For this review, take the finished solid that the model builds, in its own axes (mm). Give positions to 0.01 mm unless a question says otherwise; leave off trailing zeros. Order: outer loops, then holes, each group sorted by start corner. A loop starts at its lowest first (then second) coordinate and runs counter-clockwise, first axis right, second up. Notation, with made-up numbers: (61.25, 62) - (97.25, 62) arc R17 ccw to (97.25, 66) - close; hole circle Ø6 at (-35, -13.5). An arc over 180 degrees is marked (long way). Use a Markdown table: item, result. Add a question column.
1) We need section D-D on z = -60. Write out the cut boundary in (x, y), then the cut area to 3 significant figures.
2) Clearance check with flat-ended pins moving along their axes: P1, Ø0.9, axis at x = 84.5, y = 1.5, coming from the -Z side; P2, Ø1, axis at x = -97.5, y = 1, coming from the +Z side; P3, Ø0.9, axis at x = 87, y = 1, coming from the +Z side; P4, Ø2.5, axis at x = -60, z = 45, coming from the +Y side. State where each tip first meets the part, or that it passes through.
3) Wall thickness on L1, parallel to X at y = 0.25, z = 61; L2, parallel to Z at x = -60, y = 2; L3, parallel to X at y = 0.7, z = 15: over which ranges is each line inside the solid? List them lowest first.
4) We need section C-C on y = 1.3. Give the number of separate pieces and of enclosed holes in the cut face, then the cut area to 3 significant figures.
5) We need section B-B on z = 83.5. Write out the cut boundary in (x, y), then the cut area to 3 significant figures.
6) We need section A-A on z = 0. Write out the cut boundary in (x, y).
```python
from build123d import *

# Parameters (mm, degrees)
BOSS_EXTRUDE1_OUTLINE_R   = 150
BOSS_EXTRUDE1_OUTLINE_R_2 = 1.55
BOSS_EXTRUDE1_OUTLINE_W   = 30
BOSS_EXTRUDE1_OUTLINE_H   = 68
BOSS_EXTRUDE1_OUTLINE_R_3 = 2.25
BOSS_EXTRUDE1_DEPTH       = 3
SKETCH3_W                 = 5
SKETCH3_H                 = 63.96
SKETCH3_W_2               = 4
SKETCH3_H_2               = 6
CUT_EXTRUDE1_DEPTH        = 10


# Read off the part's stored shape, not the designer's step: Boss-Extrude1
with BuildPart() as part:
    # Boss-Extrude1 outline → Boss-Extrude1 (new body)
    with BuildSketch(Plane(origin=(0, 0, 0), x_dir=(1, 0, 0), z_dir=(0, 1, 0))):
        Circle(BOSS_EXTRUDE1_OUTLINE_R)
        with Locations((-60, -94)):
            Circle(BOSS_EXTRUDE1_OUTLINE_R_2, mode=Mode.SUBTRACT)
        with BuildLine():
            Line((-25.85, -95.55), (-31.95, -95.55))
            ThreePointArc((-31.95, -95.55), (-33.5, -94), (-31.95, -92.45))
            Line((-31.95, -92.45), (-25.85, -92.45))
            ThreePointArc((-25.85, -92.45), (-24.3, -94), (-25.85, -95.55))
        make_face(mode=Mode.SUBTRACT)
        with Locations((-89, -71)):
            Rectangle(BOSS_EXTRUDE1_OUTLINE_W, BOSS_EXTRUDE1_OUTLINE_H, mode=Mode.SUBTRACT)
        with Locations((-60, -45)):
            Circle(BOSS_EXTRUDE1_OUTLINE_R_2, mode=Mode.SUBTRACT)
        with BuildLine():
            Line((-25.85, -46.55), (-31.95, -46.55))
            ThreePointArc((-31.95, -46.55), (-33.5, -45), (-31.95, -43.45))
            Line((-31.95, -43.45), (-25.85, -43.45))
            ThreePointArc((-25.85, -43.45), (-24.3, -45), (-25.85, -46.55))
        make_face(mode=Mode.SUBTRACT)
        with BuildLine():
            Line((25.85, -92.45), (31.95, -92.45))
            ThreePointArc((31.95, -92.45), (33.5, -94), (31.95, -95.55))
            Line((31.95, -95.55), (25.85, -95.55))
            ThreePointArc((25.85, -95.55), (24.3, -94), (25.85, -92.45))
        make_face(mode=Mode.SUBTRACT)
        with Locations((60, -94)):
            Circle(BOSS_EXTRUDE1_OUTLINE_R_2, mode=Mode.SUBTRACT)
        with BuildLine():
            Line((25.85, -43.45), (31.95, -43.45))
            ThreePointArc((31.95, -43.45), (33.5, -45), (31.95, -46.55))
            Line((31.95, -46.55), (25.85, -46.55))
            ThreePointArc((25.85, -46.55), (24.3, -45), (25.85, -43.45))
        make_face(mode=Mode.SUBTRACT)
        with Locations((60, -45)):
            Circle(BOSS_EXTRUDE1_OUTLINE_R_2, mode=Mode.SUBTRACT)
        with Locations((89, -71)):
            Rectangle(BOSS_EXTRUDE1_OUTLINE_W, BOSS_EXTRUDE1_OUTLINE_H, mode=Mode.SUBTRACT)
        with Locations((-75, 85)):
            Circle(BOSS_EXTRUDE1_OUTLINE_R_3, mode=Mode.SUBTRACT)
        with Locations((75, 85)):
            Circle(BOSS_EXTRUDE1_OUTLINE_R_3, mode=Mode.SUBTRACT)
    extrude(amount=BOSS_EXTRUDE1_DEPTH)

    # Sketch3 → Cut-Extrude1 (cut)
    with BuildSketch(Plane(origin=(0, 3, 0), x_dir=(1, 0, 0), z_dir=(0, 1, 0))):
        with Locations((-26.17, 13.2)):
            Rectangle(SKETCH3_W, SKETCH3_H)
        with Locations((-26.67, 73.66)):
            Rectangle(SKETCH3_W_2, SKETCH3_H_2)
        with Locations((26.67, 73.66)):
            Rectangle(SKETCH3_W_2, SKETCH3_H_2)
        with Locations((26.17, 13.2)):
            Rectangle(SKETCH3_W, SKETCH3_H)
    extrude(amount=-CUT_EXTRUDE1_DEPTH, mode=Mode.SUBTRACT)


solid = part.part
```
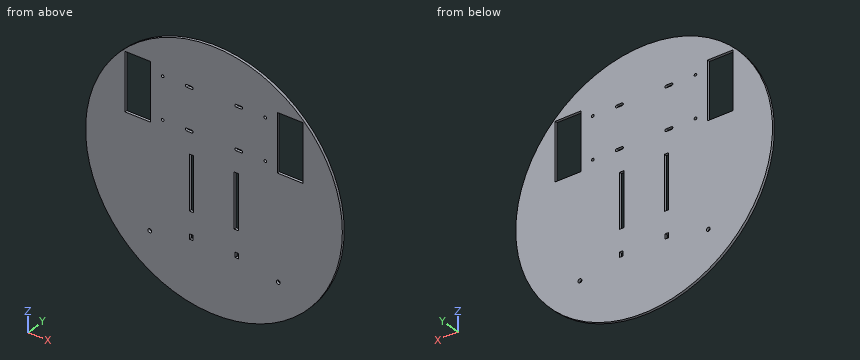
Checked values:
| question | item | result |
|---|---|---|
| 1 | outline | (-137.48, 0) - (137.48, 0) - (137.48, 3) - (-137.48, 3) - close |
| 1 | area | 825 mm² |
| 2 | P1 | z = -124.24 |
| 2 | P2 | z = 114.42 |
| 2 | P3 | z = 122.51 |
| 2 | P4 | through |
| 3 | L1 | -137.04 to -104, -74 to 74, 104 to 137.04 |
| 3 | L2 | -137.48 to 43.45, 46.55 to 92.45, 95.55 to 137.48 |
| 3 | L3 | -149.25 to -28.67, -23.67 to 23.67, 28.67 to 149.25 |
| 4 | separate pieces | 1 |
| 4 | enclosed holes | 16 |
| 4 | area | 65,800 mm² |
| 5 | outline | (-124.61, 0) - (-104, 0) - (-104, 3) - (-124.61, 3) - close; (-74, 0) - (74, 0) - (74, 3) - (-74, 3) - close; (104, 0) - (124.61, 0) - (124.61, 3) - (104, 3) - close |
| 5 | area | 568 mm² |
| 6 | outline | (-150, 0) - (-28.67, 0) - (-28.67, 3) - (-150, 3) - close; (-23.67, 0) - (23.67, 0) - (23.67, 3) - (-23.67, 3) - close; (28.67, 0) - (150, 0) - (150, 3) - (28.67, 3) - close |
